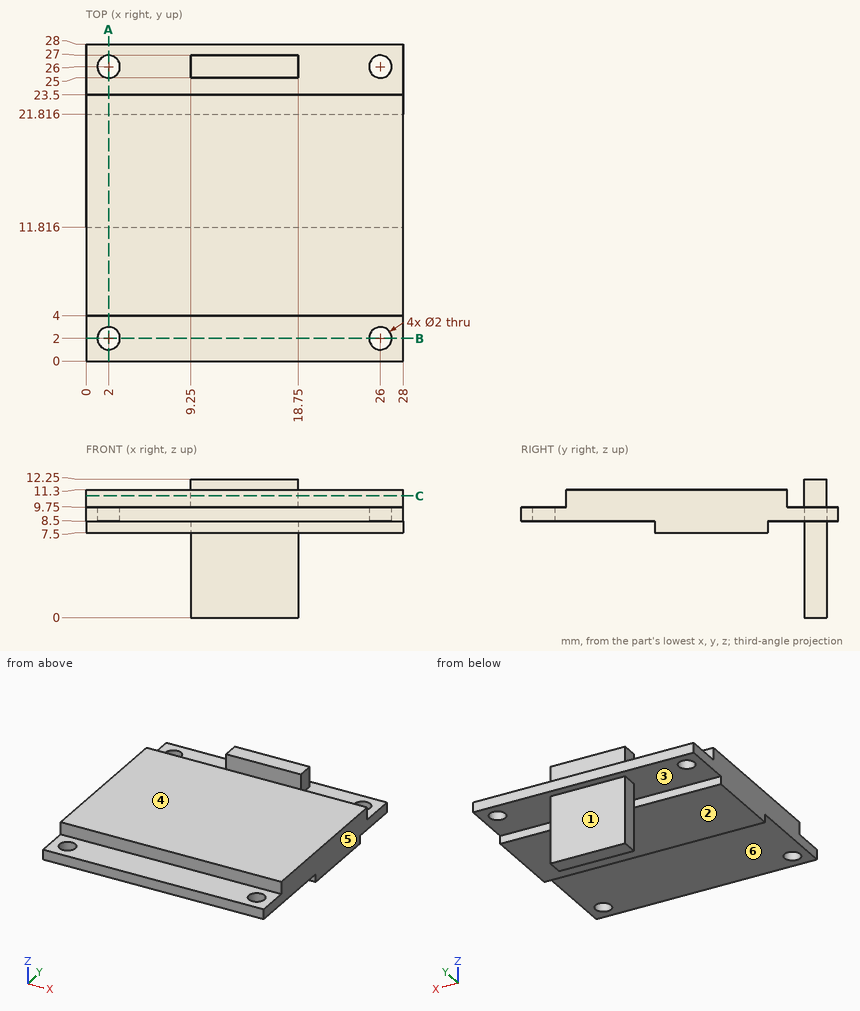
For this review, use the dimensioned drawing (mm, ordinates from the lowest corner) and the shaded views. A direction names the side the tool comes from. Give positions to 0.01 mm unless a question says otherwise; leave off trailing zeros. Loops run counter-clockwise (first coordinate to the right, second up) from the corner with the lowest first, then second, coordinate; pieces in that order, holes last.
Item 1: Insertion check: pin 1 (1.6 mm diameter, centred on y = 26, z = 11, fed in from -X); pin 2 (5 mm diameter, centred on x = 21.5, y = 8.5, fed in from +Z); pin 3 (3.5 mm diameter, centred on x = 9, y = 25.5, fed in from +Z); pin 4 (7 mm diameter, centred on x = 12.5, z = 4, fed in from +Y). Each pin has a flat end and moves straight along its axis. Give the tip position at first contact, or say it passes through.
Item 2: For line 1 along Y through (x, z) = (2, 9.1); line 2 along X through (y, z) = (26.25, 9.5); line 3 along Z through (x, y) = (23.5, 3.5), list the stretches that pass through material, from the lowest coordinate up.
Item 3: Take a section at A-A, the plane x = 2. Give the number of separate pieces and of enclosed holes in the cut face.
Item 4: Draft analysis for pull direction Y (two halves, no side actions). For the marked faces 1, 2 and 3, state which applies: +Y half, -Y half, draft (parallel to the pull), parting line (faces both ways), or undercut.
Item 5: Tool access review of the marked faces 4, 5 and 6: name each direction out of +Z, -Z, +X, -X, +Y, -Y from which nothing blocks a thin tool from reaching the whole face with its end or side.
Item 6: Take a section at B-B, the plane y = 2. State the section outline as (x, z) points.
Item 7: Take a section at C-C, the plane z = 10.75. State the section outline as (x, y) points, and give its area (3 significant figures).
Calculated:
1. pin 1: stops at x = 9.25
1. pin 2: stops at z = 11.3
1. pin 3: stops at z = 12.25
1. pin 4: stops at y = 27
2. line 1: y = 0 to 1, 3 to 25, 27 to 28
2. line 2: x = 0 to 1.03, 2.97 to 25.03, 26.97 to 28
2. line 3: z = 8.5 to 9.75
3. separate pieces: 3
3. enclosed holes: 0
4. face 1: +Y half
4. face 2: draft
4. face 3: undercut
5. face 4: +Z, +X, -X, -Y
5. face 5: +Z, -Z, +X, +Y, -Y
5. face 6: -Z, +X, -X, -Y
6. outline: (0, 8.5) - (1, 8.5) - (1, 9.75) - (0, 9.75) - close; (3, 8.5) - (25, 8.5) - (25, 9.75) - (3, 9.75) - close; (27, 8.5) - (28, 8.5) - (28, 9.75) - (27, 9.75) - close
7. outline: (0, 4) - (28, 4) - (28, 23.5) - (0, 23.5) - close; (9.25, 25) - (18.75, 25) - (18.75, 27) - (9.25, 27) - close
7. area: 565 mm2
